```python
from build123d import *

# Parameters (mm, degrees)
F0_W      = 101.6
F0_H      = 25.4
F1_DEPTH  = 12.7
F3_DEPTH  = 12.7
F4_R      = 6.35
F5_DEPTH  = 12.7
F7_R      = 12.7
F8_DEPTH  = 38.1
F9_R      = 6.9951982556
F10_DEPTH = 50.8


# Not quite as in the source:
# - ends of sketch curves that miss each other by under 0.0002 mm in the source are joined


with BuildPart() as f1:
    # F0 (on Right) → F1 (new body)
    with BuildSketch(Plane.YZ):
        with Locations((50.8, 12.7)):
            Rectangle(F0_W, F0_H)
    extrude(amount=F1_DEPTH)

    # F2 (on face) → F3 (cut)
    with BuildSketch(Plane.YZ.offset(12.7)):
        with BuildLine():
            Line((0, 25.4), (0, 12.7))
            ThreePointArc((0, 12.7), (3.7197438789, 21.6802561211), (12.7, 25.4))
            Line((12.7, 25.4), (0, 25.4))
        make_face()
        with BuildLine():
            Line((0, 0), (12.7, 0))
            ThreePointArc((12.7, 0), (3.7197438789, 3.7197438789), (0, 12.7))
            Line((0, 12.7), (0, 0))
        make_face()
        with BuildLine():
            ThreePointArc((88.9, 25.4), (97.8802564546, 21.6802563035), (101.6000005159, 12.7))
            Line((101.6000005159, 12.7), (101.6, 25.4))
            Line((101.6, 25.4), (88.9, 25.4))
        make_face()
        with BuildLine():
            ThreePointArc((101.6000005159, 12.7), (97.8802568194, 3.7197440613), (88.9000010318, 0))
            Line((88.9000010318, 0), (101.6, 0))
            Line((101.6, 0), (101.6000005159, 12.7))
        make_face()
    extrude(amount=-F3_DEPTH, mode=Mode.SUBTRACT)

    # F4 (on face) → F5 (cut)
    with BuildSketch(Plane.YZ.offset(12.7)):
        with Locations((12.7, 12.7)):
            Circle(F4_R)
        with BuildLine():
            ThreePointArc((63.5000005159, 6.35), (67.9901285764, 8.2098719395), (69.8500005159, 12.7))
            ThreePointArc((69.8500005159, 12.7), (67.9901285764, 17.1901280605), (63.5000005159, 19.05))
            ThreePointArc((63.5000005159, 19.05), (57.1500005159, 12.7), (63.5000005159, 6.35))
        make_face()
        with BuildLine():
            ThreePointArc((63.5000005159, 19.05), (67.9901285764, 17.1901280605), (69.8500005159, 12.7))
            ThreePointArc((69.8500005159, 12.7), (67.9901285764, 8.2098719395), (63.5000005159, 6.35))
            Line((63.5000005159, 6.35), (88.9000005159, 6.35))
            ThreePointArc((88.9000005159, 6.35), (82.5500005159, 12.7), (88.9000005159, 19.05))
            Line((88.9000005159, 19.05), (63.5000005159, 19.05))
        make_face()
        with BuildLine():
            ThreePointArc((95.2500005159, 12.7), (93.3901285764, 17.1901280605), (88.9000005159, 19.05))
            ThreePointArc((88.9000005159, 19.05), (82.5500005159, 12.7), (88.9000005159, 6.35))
            ThreePointArc((88.9000005159, 6.35), (93.3901285764, 8.2098719395), (95.2500005159, 12.7))
        make_face()
    extrude(amount=-F5_DEPTH, mode=Mode.SUBTRACT)

    # F7 (on face) → F8 (join)
    with BuildSketch(Plane.YZ.offset(12.7)):
        with Locations((38.1, 12.7)):
            Circle(F7_R)
    extrude(amount=F8_DEPTH)

    # F9 (on face) → F10 (cut)
    with BuildSketch(Plane.YZ.offset(50.8)):
        with Locations((38.1, 12.7)):
            Circle(F9_R)
    extrude(amount=-F10_DEPTH, mode=Mode.SUBTRACT)


solid = f1.part
```
CAD build for the part. Positions are in the model's coordinates, mm. A direction names the side the tool comes from. Round coordinates to 2 decimals unless told otherwise and drop trailing zeros. Loops run counter-clockwise (first coordinate to the right, second up) from the corner with the lowest first, then second, coordinate; pieces in that order, holes last. Notation, with made-up numbers: (53.25, 2) - (59.25, 2) arc R14 cw to (59.25, 23) - close; hole circle Ø1 at (19.25, 61). An arc over 180 degrees is marked (long way). Return JSON: item names as keys, results as strings. Group by question number.
Q1. Band-saw the part on B-B on x = 4.5. Give the cut face in (y, z).
Q2. Drill centre lines: line 1 along Z through (x, y) = (20, 38); line 2 along Y through (x, z) = (11, 7.5); line 3 along Y through (x, z) = (21, 13). Where is each one in solid material? Low to high. Write a range as [from, to].
Q3. Flat gauge pins, fed straight in: pin 1 Ø10 at (x, y) = (25, 52) entering from +Z; pin 2 Ø1 at (x, z) = (15, 21.5) entering from +Y; pin 3 Ø1.5 at (x, z) = (27, 12) entering from -Y. Where does each tip first touch, or does it go through?
Q4. Band-saw the part on C-C on z = 15.5. Give the cut face in (x, y), plus the area to 3 significant figures.
Q5. Band-saw the part on D-D on x = 36. Give the cut face in (y, z).
Q6. Tool access for faces 1 (the face through (6, 76, 6.35)), 2 (the face through (6, 50, 25.4)): list every direction of +Z, -Z, +X, -X, +Y, -Y with a clear straight run to the whole face (end or side of a thin tool).
Q7. Band-saw the part on A-A on y = 59. Give the cut face in (x, z).
Q8. Two-plate mould, pull along Z, no slides. Class faces 3 (the face through (6, 76, 19.05)), 4 (the face through (31.483, 50.214, 16.515)), 5 (the face through (6, 50, 0)), 6 (the face through (0, 50, 13)): +Z half, -Z half, draft (parallel to the pull), parting line (faces both ways), or undercut.
Solutions:
{
 "1": {"outline": "(12.7, 0) - (88.9, 0) arc R12.7 ccw to (88.9, 25.4) - (12.7, 25.4) arc R12.7 ccw to start; hole circle Ø12.7 at (12.7, 12.7); hole circle Ø13.99 at (38.1, 12.7); hole (63.5, 6.35) - (88.9, 6.35) arc R6.35 ccw to (88.9, 19.05) - (63.5, 19.05) arc R6.35 ccw to start"},
 "2": {"line 1": "z = [0, 5.71], [19.69, 25.4]", "line 2": "y = [1.11, 9.06], [16.34, 33.42], [42.78, 59.86], [92.54, 100.49]", "line 3": "y = [25.4, 31.11], [45.09, 50.8]"},
 "3": {"pin 1": "stops at z = 21.76", "pin 2": "stops at y = 47.71", "pin 3": "stops at y = 25.4"},
 "4": {"outline": "(0, 0.31) - (12.7, 0.31) - (12.7, 7) - (0, 7) - close; (0, 18.4) - (12.7, 18.4) - (12.7, 25.71) - (50.8, 25.71) - (50.8, 31.69) - (0, 31.69) - close; (0, 44.51) - (50.8, 44.51) - (50.8, 50.49) - (12.7, 50.49) - (12.7, 57.8) - (0, 57.8) - close; (0, 94.6) - (12.7, 94.6) - (12.7, 101.29) - (0, 101.29) - close", "area": "963 mm^2"},
 "5": {"outline": "circle Ø25.4 at (38.1, 12.7); hole circle Ø13.99 at (38.1, 12.7)"},
 "6": {"face 1": "+X, -X", "face 2": "+Z, +X, -X, +Y, -Y"},
 "7": {"outline": "(0, 0) - (12.7, 0) - (12.7, 8.22) - (0, 8.22) - close; (0, 17.18) - (12.7, 17.18) - (12.7, 25.4) - (0, 25.4) - close"},
 "8": {"face 3": "undercut", "face 4": "parting line", "face 5": "-Z half", "face 6": "draft"}
}
